The listing builds one solid part. Answer for the finished solid, in the listing's coordinates (mm). A direction names the side the tool comes from. Coordinates: 2 decimals unless noted, no trailing zeros. Order: outer loops, then holes, each group sorted by start corner. A loop starts at its lowest first (then second) coordinate and runs counter-clockwise, first axis right, second up. Notation, with made-up numbers: (-18.75, -14) -> (11.25, -14) arc R15 ccw to (11.25, -5) -> close; hole circle Ø7 at (37, 70.25). An arc over 180 degrees is marked (long way). Answer in a Markdown table with one row per item.
```python
from build123d import *

# Parameters (mm, degrees)
F0_W     = 25
F0_H     = 15
F1_DEPTH = 4
F2_R     = 5
F3_DEPTH = 1.5
F5_DEPTH = 80
F6_SIZE  = 1
F8_DEPTH = 25


with BuildPart() as f1:
    # F0 (on Front) → F1 (new body)
    with BuildSketch(Plane.XZ):
        Rectangle(F0_W, F0_H)
    extrude(amount=F1_DEPTH)

    # F2 (on Front) → F3 (cut)
    with BuildSketch(Plane.XZ):
        Circle(F2_R)
    extrude(amount=F3_DEPTH, mode=Mode.SUBTRACT)

    # F4 (on face) → F5 (join)
    with BuildSketch(Plane.XZ.offset(4)):
        Polygon((4, 7.5), (0, 7.5), (-4, 7.5), (-4, 3.5), (4, 3.5), align=None)
    extrude(amount=F5_DEPTH)

    # F6
    f6_edges = [f1.edges().sort_by_distance(p)[0] for p in [
        (8.25, -4, 7.5),
        (-8.25, -4, 7.5),
        (-12.5, -4, 0),
        (0, -4, -7.5),
        (12.5, -4, 0),
    ]]
    chamfer(f6_edges, length=F6_SIZE)

    # F7 (on face) → F8 (cut)
    with BuildSketch(Plane.XZ.offset(4)):
        with BuildLine():
            ThreePointArc((13.912691, 7.559422), (11.895218, 8.876943), (11.5, 6.5))
            ThreePointArc((11.5, 6.5), (13.052276, 6.241901), (13.912691, 7.559422))
        make_face()
        with BuildLine():
            ThreePointArc((-11.5, 6.5), (-11.196021, 6.959825), (-11.089372, 7.500628))
            ThreePointArc((-11.089372, 7.500628), (-13.831705, 8.041431), (-11.5, 6.5))
        make_face()
    extrude(amount=-F8_DEPTH, mode=Mode.SUBTRACT)


solid = f1.part
```
(1) Flat-ended cylindrical pins translate along their axes: pin 1 (12 mm diameter, centred on x = -9.5, y = -57, fed in from -Z); pin 2 (8 mm diameter, centred on x = 0.5, z = 1, fed in from +Y); pin 3 (1 mm diameter, centred on y = -47.5, z = 1.5, fed in from -X); pin 4 (1.2 mm diameter, centred on y = -33.5, z = 5, fed in from -X). Find the tip coordinate at first contact, or state that the pin passes through.
Check values:
| item | result |
|---|---|
| pin 1 | z = 3.5 |
| pin 2 | y = 0 |
| pin 3 | through |
| pin 4 | x = -4 |
(2) A cutting plane is placed at C-C, the plane y = -60.5. Determine the outline of the cut face in (x, z), then the cut area to 3 significant figures.
Check values:
| item | result |
|---|---|
| outline | (-4, 3.5) -> (4, 3.5) -> (4, 7.5) -> (-4, 7.5) -> close |
| area | 32.0 mm² |
(3) For a pull along Z with two mould halves and no side action, classify faces 1 (the cylindrical face through (-1.08, -0.74, -4.88)), 2 (the flat face through (0, -39, 7.5)), 3 (the flat face through (4, -43, 5)) as released by +Z, released by -Z, zero draft, split by the parting line, or undercut.
Check values:
| item | result |
|---|---|
| face 1 | undercut |
| face 2 | released by +Z |
| face 3 | zero draft |
(4) A cutting plane is placed at D-D, the plane x = 0. Determine the outline of the cut face in (y, z).
Check values:
| item | result |
|---|---|
| outline | (-84, 3.5) -> (-4, 3.5) -> (-4, -6.5) -> (-3, -7.5) -> (0, -7.5) -> (0, -5) -> (-1.5, -5) -> (-1.5, 5) -> (0, 5) -> (0, 7.5) -> (-84, 7.5) -> close |
(5) Which of the six approach directions +Z, -Z, +X, -X, +Y, -Y give full straight-line access (tool end or side, diameter ignored) to faces 4 (the flat face through (0, -1.5, 0)), 5 (the flat face through (-12.5, -1, -1)), 6 (the flat face through (0, -43, 3.5))?
Check values:
| item | result |
|---|---|
| face 4 | +Y |
| face 5 | +Z, -Z, -X, +Y, -Y |
| face 6 | -Z, +X, -X, -Y |
(6) A cutting plane is placed at A-A, the plane x = 9.75. Determine the outline of the cut face in (y, z).
Check values:
| item | result |
|---|---|
| outline | (-4, -6.5) -> (-3, -7.5) -> (0, -7.5) -> (0, 7.5) -> (-3, 7.5) -> (-4, 6.5) -> close |
(7) A cutting plane is placed at B-B, the plane z = 0. Determine the outline of the cut face in (x, y), then the cut area to 3 significant figures.
Check values:
| item | result |
|---|---|
| outline | (-12.5, -3) -> (-11.5, -4) -> (11.5, -4) -> (12.5, -3) -> (12.5, 0) -> (5, 0) -> (5, -1.5) -> (-5, -1.5) -> (-5, 0) -> (-12.5, 0) -> close |
| area | 84.0 mm² |
(8) Find the intervals of material crossed by line 1 along Z through (x, y) = (0, -0.85); line 2 along Y through (x, z) = (-2.75, -5.5); line 3 along Z through (x, y) = (-0.5, -70.5), in increasing order. Write a range as from..to.
Check values:
| item | result |
|---|---|
| line 1 | -7.5..-5, 5..7.5 |
| line 2 | -4..0 |
| line 3 | 3.5..7.5 |
